from build123d import *

# Parameters (mm, degrees)
F0_R     = 127
F0_R_2   = 6.35
F1_DEPTH = 6.35
F2_R     = 3.175
F3_DEPTH = 203.2


with BuildPart() as f1:
    # F0 (on Front) → F1 (new body)
    with BuildSketch(Plane.XZ):
        Circle(F0_R)
        Circle(F0_R_2, mode=Mode.SUBTRACT)
    extrude(amount=F1_DEPTH)

    # F2 (on face) → F3 (join)
    with BuildSketch(Plane.XZ.offset(6.35)):
        with Locations((114.3, 0)):
            Circle(F2_R)
        with Locations((-57.15, 98.986704)):
            Circle(F2_R)
        with Locations((-57.15, -98.986704)):
            Circle(F2_R)
    extrude(amount=F3_DEPTH)


solid = f1.part
For this review, take the finished solid that the model builds, in its own axes (mm). A direction names the side the tool comes from. Give positions to 0.01 mm unless a question says otherwise; leave off trailing zeros. Order: outer loops, then holes, each group sorted by start corner. A loop starts at its lowest first (then second) coordinate and runs counter-clockwise, first axis right, second up. Notation, with made-up numbers: (71.5, 63) - (75.5, 63) arc R7 cw to (75.5, 69) - close; hole circle Ø8 at (0.5, 9). An arc over 180 degrees is marked (long way). Answer as a JSON object with one key per item and string values. Group by question number.
Item 1: Draft analysis for pull direction Z (two halves, no side actions). For faces 1 (the flat face through (114, -209.55, 0)), 2 (the cylindrical face through (-55.44, -106.53, 101.66)), 3 (the cylindrical face through (117.33, -106.53, 0.95)), state which applies: pulls with the +Z half, pulls with the -Z half, needs draft (parallel to the pull), parting line crosses it, or undercut.
Item 2: Take a section at B-B on y = -121. Give the boundary of the cut face in (x, z) (3 decimals).
Item 3: Take a section at A-A on x = 0. Give the boundary of the cut face in (y, z), and give its area (3 significant figures).
Item 4: Wall thickness on line 1 along Z through (x, y) = (0, -3.75); line 2 along Y through (x, z) = (-3.5, 90); line 3 along Z through (x, y) = (-59, -72): over which ranges is each line inside the solid? List them lowest first.
Item 5: Take a section at D-D on x = 93. Give the boundary of the cut face in (y, z), and give its area (3 significant figures).
Item 6: Clearance check with flat-ended pins moving along their axes: pin 1 Ø11.5 at (x, z) = (0, 0) entering from -Y; pin 2 Ø1 at (x, z) = (-94.5, 29.5) entering from -Y. State where each tip first meets the part, or that it passes through.
Item 7: Take a section at C-C on z = -68. Give the boundary of the cut face in (x, y).
Item 8: Machinability: for faces 4 (the cylindrical face through (-27.53, -3.13, -123.98)), 5 (the cylindrical face through (-55.44, -106.53, -96.31)), which of the approach directions +Z, -Z, +X, -X, +Y, -Y give a long, thin tool a straight path to every point of the face, cutting with its end or side? Answer none if there is none.
Reported:
{
 "1": {"face 1": "needs draft", "face 2": "undercut", "face 3": "parting line crosses it"},
 "2": {"outline": "circle Ø6.35 at (-57.15, -98.987); circle Ø6.35 at (-57.15, 98.987); circle Ø6.35 at (114.3, 0)"},
 "3": {"outline": "(-6.35, -127) - (0, -127) - (0, -6.35) - (-6.35, -6.35) - close; (-6.35, 6.35) - (0, 6.35) - (0, 127) - (-6.35, 127) - close", "area": "1,530 mm^2"},
 "4": {"line 1": "-127 to -6.35, 6.35 to 127", "line 2": "-6.35 to 0", "line 3": "-101.57 to -96.41, 96.41 to 101.57"},
 "5": {"outline": "(-6.35, -86.49) - (0, -86.49) - (0, 86.49) - (-6.35, 86.49) - close", "area": "1,100 mm^2"},
 "6": {"pin 1": "through", "pin 2": "y = -6.35"},
 "7": {"outline": "(-107.26, -6.35) - (107.26, -6.35) - (107.26, 0) - (-107.26, 0) - close"},
 "8": {"face 4": "+Y, -Y", "face 5": "-Y"}
}
